```python
from build123d import *

# Parameters (mm, degrees)
SKETCH_1_W             = 23.5
SKETCH_1_H             = 12
EXTRUDE_1_DEPTH        = 771
HOLE_WIZARD_M6_3_D     = 5
HOLE_WIZARD_M6_3_DEPTH = 15
HOLE_WIZARD_M6_3_TIP   = 1.502151548
SKETCH_13_R            = 5.05
CUT_EXTRUDE_6_DEPTH    = 772.729227126
HOLE_WIZARD_M6_4_D     = 5
HOLE_WIZARD_M6_4_DEPTH = 15
HOLE_WIZARD_M6_4_TIP   = 1.502151548
SKETCH_10_R            = 4.5
CUT_EXTRUDE_7_DEPTH    = 772.729227126
HOLE_WIZARD_M6_5_D     = 5
HOLE_WIZARD_M6_5_DEPTH = 15
HOLE_WIZARD_M6_5_TIP   = 1.502151548


with BuildPart() as part:
    # 草图1 → 凸台-拉伸1 (new, symmetric)
    with BuildSketch(Plane(origin=(0, 0, 0), x_dir=(0, 0, -1), z_dir=(1, 0, 0))):
        with BuildLine():
            Line((-14, 15), (-11.5, 15))
            Line((-11.5, 15), (-11.5, 13.5))
            Line((-11.5, 13.5), (-11.4, 13.5))
            ThreePointArc((-11.4, 13.5), (-11.117157288, 13.382842712), (-11, 13.1))
            Line((-11, 13.1), (-11, 12))
            Line((-11, 12), (-9.5, 12))
            Line((-9.5, 12), (-9.5, 15))
            Line((-9.5, 15), (-8, 15))
            Line((-8, 15), (-8, 12.5))
            Line((-8, 12.5), (-5, 12.5))
            Line((-5, 12.5), (-5, 15))
            Line((-5, 15), (5, 15))
            Line((5, 15), (5, 12.5))
            Line((5, 12.5), (8, 12.5))
            Line((8, 12.5), (8, 15))
            Line((8, 15), (9.5, 15))
            Line((9.5, 15), (9.5, 12))
            Line((9.5, 12), (11, 12))
            Line((11, 12), (11, 13.1))
            ThreePointArc((11, 13.1), (11.117157288, 13.382842712), (11.4, 13.5))
            Line((11.4, 13.5), (11.5, 13.5))
            Line((11.5, 13.5), (11.5, 15))
            Line((11.5, 15), (14, 15))
            ThreePointArc((14, 15), (14.707106781, 14.707106781), (15, 14))
            Line((15, 14), (15, 8))
            Line((15, 8), (12.5, 8))
            Line((12.5, 8), (12.5, 5))
            Line((12.5, 5), (15, 5))
            Line((15, 5), (15, -5))
            Line((15, -5), (12.5, -5))
            Line((12.5, -5), (12.5, -8))
            Line((12.5, -8), (15, -8))
            Line((15, -8), (15, -14))
            ThreePointArc((15, -14), (14.707106781, -14.707106781), (14, -15))
            Line((14, -15), (11.5, -15))
            Line((11.5, -15), (11.5, -13.5))
            Line((11.5, -13.5), (11.4, -13.5))
            ThreePointArc((11.4, -13.5), (11.117157288, -13.382842712), (11, -13.1))
            Line((11, -13.1), (11, -12))
            Line((11, -12), (9.5, -12))
            Line((9.5, -12), (9.5, -15))
            Line((9.5, -15), (8, -15))
            Line((8, -15), (8, -12.5))
            Line((8, -12.5), (5, -12.5))
            Line((5, -12.5), (5, -15))
            Line((5, -15), (-5, -15))
            Line((-5, -15), (-5, -12.5))
            Line((-5, -12.5), (-8, -12.5))
            Line((-8, -12.5), (-8, -15))
            Line((-8, -15), (-9.5, -15))
            Line((-9.5, -15), (-9.5, -12))
            Line((-9.5, -12), (-11, -12))
            Line((-11, -12), (-11, -13.1))
            ThreePointArc((-11, -13.1), (-11.117157288, -13.382842712), (-11.4, -13.5))
            Line((-11.4, -13.5), (-11.5, -13.5))
            Line((-11.5, -13.5), (-11.5, -15))
            Line((-11.5, -15), (-14, -15))
            ThreePointArc((-14, -15), (-14.707106781, -14.707106781), (-15, -14))
            Line((-15, -14), (-15, 14))
            ThreePointArc((-15, 14), (-14.707106781, 14.707106781), (-14, 15))
        make_face()
        with BuildLine():
            Line((12, -10.5), (12, -8.5))
            ThreePointArc((12, -8.5), (11.853553391, -8.146446609), (11.5, -8))
            Line((11.5, -8), (-11.5, -8))
            ThreePointArc((-11.5, -8), (-11.853553391, -8.146446609), (-12, -8.5))
            Line((-12, -8.5), (-12, -10.5))
            ThreePointArc((-12, -10.5), (-11.853553391, -10.853553391), (-11.5, -11))
            Line((-11.5, -11), (11.5, -11))
            ThreePointArc((11.5, -11), (11.853553391, -10.853553391), (12, -10.5))
        make_face(mode=Mode.SUBTRACT)
        with BuildLine():
            Line((-11.5, 11), (11.5, 11))
            ThreePointArc((11.5, 11), (11.853553391, 10.853553391), (12, 10.5))
            Line((12, 10.5), (12, 8.5))
            ThreePointArc((12, 8.5), (11.853553391, 8.146446609), (11.5, 8))
            Line((11.5, 8), (-11.5, 8))
            ThreePointArc((-11.5, 8), (-11.853553391, 8.146446609), (-12, 8.5))
            Line((-12, 8.5), (-12, 10.5))
            ThreePointArc((-12, 10.5), (-11.853553391, 10.853553391), (-11.5, 11))
        make_face(mode=Mode.SUBTRACT)
        Rectangle(SKETCH_1_W, SKETCH_1_H, mode=Mode.SUBTRACT)
    extrude(amount=EXTRUDE_1_DEPTH, both=True)

    # M6 螺纹孔3
    with Locations(Plane(origin=(0, 0, -15), x_dir=(-1, 0, 0), z_dir=(0, 0, -1))):
        with Locations((-751, 0), (-736, 0), (736, 0), (751, 0)):
            Hole(HOLE_WIZARD_M6_3_D / 2, depth=HOLE_WIZARD_M6_3_DEPTH)
            with Locations((0, 0, -(HOLE_WIZARD_M6_3_DEPTH + HOLE_WIZARD_M6_3_TIP / 2))):  # 118° drill point
                Cone(0, HOLE_WIZARD_M6_3_D / 2, HOLE_WIZARD_M6_3_TIP, mode=Mode.SUBTRACT)

    # 草图13 → 切除-拉伸6 (cut, through all)
    with BuildSketch(Plane(origin=(0, 0, -15), x_dir=(-1, 0, 0), z_dir=(0, 0, -1))):
        Circle(SKETCH_13_R)
        with Locations((25, 0)):
            Circle(SKETCH_13_R)
        with Locations((-25, 0)):
            Circle(SKETCH_13_R)
    extrude(amount=-CUT_EXTRUDE_6_DEPTH, mode=Mode.SUBTRACT)

    # M6 螺纹孔4
    with Locations(Plane(origin=(0, 0, -15), x_dir=(-1, 0, 0), z_dir=(0, 0, -1))):
        with Locations((-411, 0), (-351, 0), (351, 0), (411, 0)):
            Hole(HOLE_WIZARD_M6_4_D / 2, depth=HOLE_WIZARD_M6_4_DEPTH)
            with Locations((0, 0, -(HOLE_WIZARD_M6_4_DEPTH + HOLE_WIZARD_M6_4_TIP / 2))):  # 118° drill point
                Cone(0, HOLE_WIZARD_M6_4_D / 2, HOLE_WIZARD_M6_4_TIP, mode=Mode.SUBTRACT)

    # 草图10 → 切除-拉伸7 (cut, through all)
    with BuildSketch(Plane(origin=(0, 0, -15), x_dir=(-1, 0, 0), z_dir=(0, 0, -1))):
        with Locations((-651, 0)):
            Circle(SKETCH_10_R)
        with Locations((-221, 0)):
            Circle(SKETCH_10_R)
        with Locations((221, 0)):
            Circle(SKETCH_10_R)
        with Locations((651, 0)):
            Circle(SKETCH_10_R)
        with Locations((691, 0)):
            Circle(SKETCH_10_R)
        with Locations((-691, 0)):
            Circle(SKETCH_10_R)
    extrude(amount=-CUT_EXTRUDE_7_DEPTH, mode=Mode.SUBTRACT)

    # M6 螺纹孔5
    with Locations(Plane(origin=(0, 15, 0), x_dir=(-1, 0, 0), z_dir=(0, 1, 0))):
        with Locations((-751, 0), (-736, 0), (736, 0), (751, 0)):
            Hole(HOLE_WIZARD_M6_5_D / 2, depth=HOLE_WIZARD_M6_5_DEPTH)
            with Locations((0, 0, -(HOLE_WIZARD_M6_5_DEPTH + HOLE_WIZARD_M6_5_TIP / 2))):  # 118° drill point
                Cone(0, HOLE_WIZARD_M6_5_D / 2, HOLE_WIZARD_M6_5_TIP, mode=Mode.SUBTRACT)


solid = part.part
```
The listing builds one solid part. Answer for the finished solid, in the listing's coordinates (mm). Give positions to 0.01 mm unless a question says otherwise; leave off trailing zeros. Return JSON: item names as keys, results as strings. Group by question number.
1. Straight lines are drawn through the part: line 1 (Y direction, x = -583, z = 0.5); line 2 (Y direction, x = 751, z = -13); line 3 (Y direction, x = 651, z = 12.95). For each, find the intervals that lie inside material, in ascending order. Write a range as [from, to].
2. Determine the mould class of faces 1 (the flat face through (11, 6, 0)), 2 (the flat face through (11, -6, 0)), 3 (the flat face through (771, 7, 0)) for opening direction Y: pulls with the +Y half, pulls with the -Y half, needs draft (parallel to the pull), parting line crosses it, or undercut.
3. Given pin 1 Ø1.5 at (x, z) = (-509, -6) entering from +Y, flat-ended and moving along its own axis, determine where the tip first touches the part or whether it passes through.
4. Find section A-A (x = 555). State how many separate pieces and enclosed holes the cut face has, then the cut area to 3 significant figures.
Verdict:
{
 "1": {"line 1": "y = [-15, -11], [-8, -6], [6, 8], [11, 15]", "line 2": "y = [-15, -8], [-5, -2.5], [2.5, 5], [8, 15]", "line 3": "y = [-15, -4.5], [4.5, 15]"},
 "2": {"face 1": "undercut", "face 2": "undercut", "face 3": "needs draft"},
 "3": {"pin 1": "stops at y = 12.5"},
 "4": {"separate pieces": "1", "enclosed holes": "3", "area": "407 mm^2"}
}
